Part print with two shaded views. Sizes in mm from the minimum x, y, z corner. Give positions to 0.01 mm unless a question says otherwise; leave off trailing zeros. Write each loop counter-clockwise with the first axis right and the second up, starting at its lowest first coordinate (ties: lowest second). Pieces come first, ordered by that corner, then holes. Notation, with made-up numbers: (25.5, -23) - (71.5, -23) arc R31 ccw to (71.5, 10) - close; hole circle Ø10 at (68, 56.5). An arc over 180 degrees is marked (long way). Answer as a JSON object with one key per item and string values.
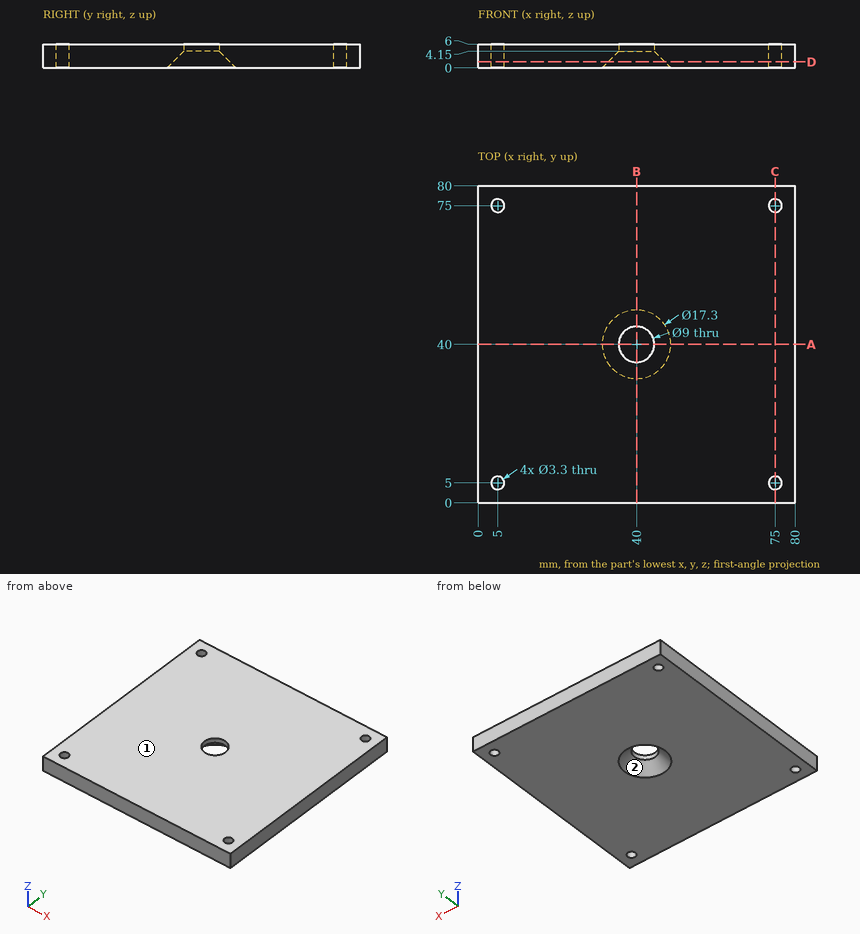
(1) Pull direction Y, two halves, no side cores. Call the marked faces 1 and 2: pulls with the +Y half, pulls with the -Y half, needs draft (parallel to the pull), parting line crosses it, or undercut.
Answer key:
{"face 1": "needs draft", "face 2": "undercut"}
(2) Probe L1, parallel to Y at x = 75, z = 3.25; L2, parallel to X at y = 40, z = 5. List the from-to ranges inside material, lowest first. Write a range as [from, to].
Answer key:
{"L1": "y = [0, 3.35], [6.65, 73.35], [76.65, 80]", "L2": "x = [0, 35.5], [44.5, 80]"}
(3) Saw through at C-C, the plane x = 75. Give the cut face in (y, z), and give its area (3 significant figures).
Answer key:
{"outline": "(0, 0) - (3.35, 0) - (3.35, 6) - (0, 6) - close; (6.65, 0) - (73.35, 0) - (73.35, 6) - (6.65, 6) - close; (76.65, 0) - (80, 0) - (80, 6) - (76.65, 6) - close", "area": "440 mm²"}
(4) Saw through at A-A, the plane y = 40. Give the cut face in (x, z), and give its area (3 significant figures).
Answer key:
{"outline": "(0, 0) - (31.35, 0) - (35.5, 4.15) - (35.5, 6) - (0, 6) - close; (44.5, 4.15) - (48.65, 0) - (80, 0) - (80, 6) - (44.5, 6) - close", "area": "409 mm²"}
(5) Saw through at D-D, the plane z = 1.5. Give the cut face in (x, y), and give its area (3 significant figures).
Answer key:
{"outline": "(0, 0) - (80, 0) - (80, 80) - (0, 80) - close; hole circle Ø3.3 at (5, 5); hole circle Ø3.3 at (5, 75); hole circle Ø14.3 at (40, 40); hole circle Ø3.3 at (75, 5); hole circle Ø3.3 at (75, 75)", "area": "6,210 mm²"}
